Input: dimensioned drawing with shaded views. Units: mm. Origin: part minimum x, y, z. A direction names the side the tool comes from. Round coordinates to 2 decimals unless told otherwise and drop trailing zeros. Loops run counter-clockwise (first coordinate to the right, second up) from the corner with the lowest first, then second, coordinate; pieces in that order, holes last. Notation, with made-up numbers: (58.25, 30.25) - (111.25, 30.25) arc R23 ccw to (111.25, 58.25) - close; hole circle Ø1 at (62.25, -4.5). An arc over 180 degrees is marked (long way). Answer as CSV lines item,"result".
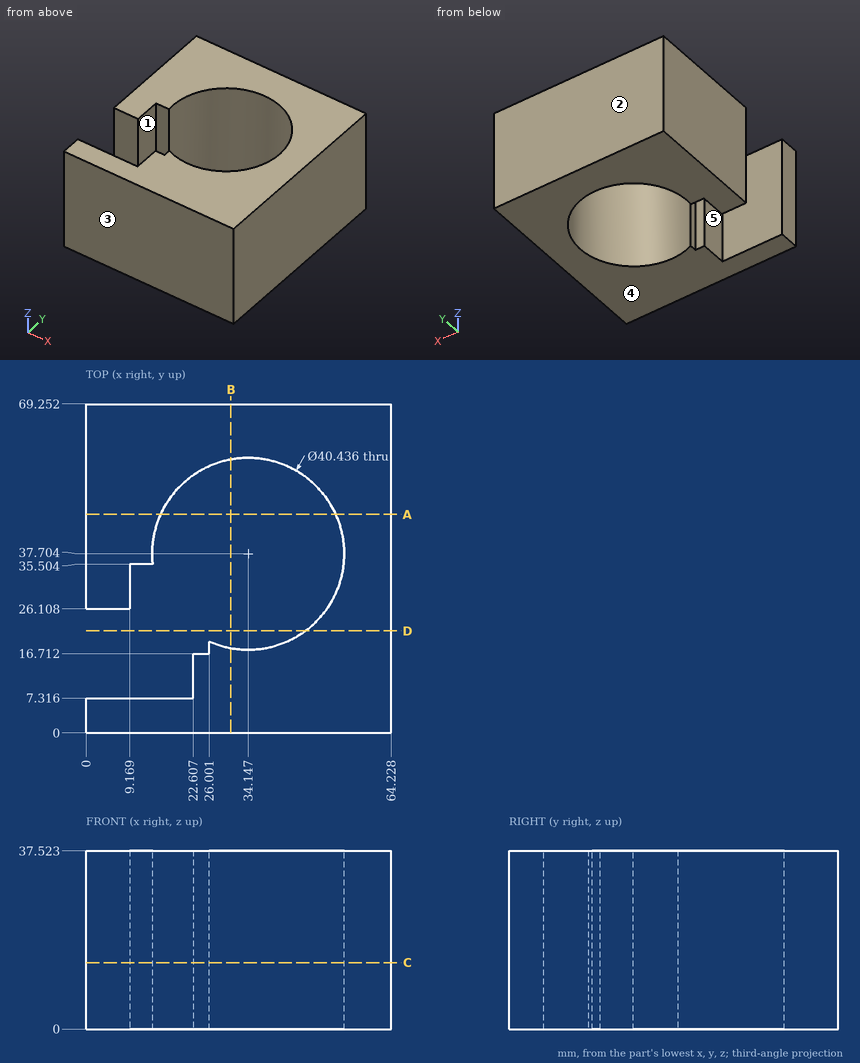
(1) Section D-D (y = 21.5). Output: boundary loops of the cut face in (x, z), and give its area (3 significant figures).
Findings below:
outline,"(46.24, 0) - (64.23, 0) - (64.23, 37.52) - (46.24, 37.52) - close"
area,"675 mm2"
(2) Section A-A (y = 46). Output: boundary loops of the cut face in (x, z) (1 decimal), and give its area (3 significant figures).
Findings below:
outline,"(0, 0) - (15.7, 0) - (15.7, 37.5) - (0, 37.5) - close; (52.6, 0) - (64.2, 0) - (64.2, 37.5) - (52.6, 37.5) - close"
area,"1,030 mm2"
(3) Pin query (flat end, axial travel): P1, Ø12, axis at x = 28, z = 20.5, coming from the -Y side; P2, Ø0.7, axis at y = 17.5, z = 23.5, coming from the -X side; P3, Ø8, axis at y = 19, z = 5.5, coming from the -X side. Return the tip coordinate at first contact, or that it passes through.
Findings below:
P1,"y = 0"
P2,"x = 26"
P3,"x = 22.61"
(4) Draft query along Y for the marked faces 1, 2 and 3. Return one class per face: pulls with the +Y half, pulls with the -Y half, needs draft (parallel to the pull), parting line crosses it, or undercut.
Findings below:
face 1,"undercut"
face 2,"pulls with the +Y half"
face 3,"pulls with the -Y half"
(5) Section B-B (x = 30.5). Output: boundary loops of the cut face in (y, z), and give its area (3 significant figures).
Findings below:
outline,"(0, 0) - (17.82, 0) - (17.82, 37.52) - (0, 37.52) - close; (57.59, 0) - (69.25, 0) - (69.25, 37.52) - (57.59, 37.52) - close"
area,"1,110 mm2"
(6) Section C-C (z = 14). Output: boundary loops of the cut face in (x, y) (1 decimal), and give its area (3 significant figures).
Findings below:
outline,"(0, 0) - (64.2, 0) - (64.2, 69.3) - (0, 69.3) - (0, 26.1) - (9.2, 26.1) - (9.2, 35.5) - (14, 35.5) arc R20.2 cw (long way) to (26, 19.2) - (26, 16.7) - (22.6, 16.7) - (22.6, 7.3) - (0, 7.3) - close"
area,"2,680 mm2"
(7) Access query for the marked faces 4 and 5. Directions: +Z, -Z, +X, -X, +Y, -Y. A direction counts if a zero-diameter tool reaches every point of the face in a straight line with its end or side. Return the directions, or none.
Findings below:
face 4,"-Z, +X, -X, +Y, -Y"
face 5,"+Z, -Z, -X"
(8) Material intervals for line 1 along Y through (x, z) = (10, 19) (1 decimal); line 2 along Y through (x, z) = (23, 6); line 3 along X through (y, z) = (41.5, 3.5) (1 decimal), sorted ascending.
Findings below:
line 1,"0 to 7.3, 35.5 to 69.3"
line 2,"0 to 16.71, 54.57 to 69.25"
line 3,"0 to 14.3, 54 to 64.2"
